from build123d import *

# Parameters (mm, degrees)
RESSALTO_EXTRUS_O1_DEPTH   = 285
CORTE_EXTRUS_O1_DEPTH      = 1
CORTE_EXTRUS_O1_DEPTH_BACK = 286


with BuildPart() as part:
    # Esboço1 → Ressalto-extrusão1 (new body)
    with BuildSketch(Plane.XY):
        Polygon((0.129363371, 0.000429576), (0.129363371, 50.000429576), (115.229363371, 50.000429576), (115.229363371, 0.000429576), (112.558897843, 0.0275034), (111.229363371, 41.700429576), (105.129363371, 41.700429576), (103.799966135, 0.000429576), (102.459761608, 0.000429576), (101.129363371, 41.700429576), (95.029363371, 41.700429576), (93.699966135, 0.000429576), (92.359761608, 0.000429576), (91.029363371, 41.700429576), (84.929363371, 41.700429576), (83.599966135, 0.000429576), (82.259761608, 0.000429576), (80.929363371, 41.700429576), (74.829363371, 41.700429576), (73.499966135, 0.000429576), (72.159761608, 0.000429576), (70.829363371, 41.700429576), (64.729363371, 41.700429576), (63.399966135, 0.000429576), (62.059761608, 0.000429576), (60.729363371, 41.700429576), (54.629363371, 41.700429576), (53.299966135, 0.000429576), (51.959761608, 0.000429576), (50.629363371, 41.700429576), (44.529363371, 41.700429576), (43.199966135, 0.000429576), (41.859761608, 0.000429576), (40.529363371, 41.700429576), (34.429363371, 41.700429576), (33.099966135, 0.000429576), (31.759761608, 0.000429576), (30.429363371, 41.700429576), (24.329363371, 41.700429576), (22.999966135, 0.000429576), (21.659761608, 0.000429576), (20.329363371, 41.700429576), (14.229363371, 41.700429576), (12.899966135, 0.000429576), (11.559761608, 0.000429576), (10.229363371, 41.700429576), (4.129363371, 41.700429576), (2.799966135, 0.000429576), align=None)
    extrude(amount=RESSALTO_EXTRUS_O1_DEPTH)

    # Esboço2 → Corte-extrusão1 (cut, two sides)
    with BuildSketch(Plane(origin=(0, 0, 0), x_dir=(-1, 0, 0), z_dir=(0, 0, -1))) as corte_extrus_o1_sk:
        Polygon((-104.72087071, 48.268772175), (-101.689781797, 46.518772175), (-102.689781797, 44.786721368), (-105.72087071, 46.536721368), (-108.513105078, 41.700429576), (-108.513105078, 0.000429576), (-115.229363371, 0.000429576), (-115.229363371, 50.000429576), (-103.74577832, 50.000429576), align=None)
        Polygon((-10.613175555, 48.268772175), (-8.881124748, 49.268772175), (-7.881124748, 47.536721368), (-9.613175555, 46.536721368), (-6.820941187, 41.700429576), (-6.820941187, 0), (0, 0), (-0.129363371, 50.000429576), (-11.612948422, 50.000429576), align=None)
    extrude(amount=CORTE_EXTRUS_O1_DEPTH, mode=Mode.SUBTRACT)
    extrude(corte_extrus_o1_sk.sketch, amount=-CORTE_EXTRUS_O1_DEPTH_BACK, mode=Mode.SUBTRACT)


solid = part.part
The listing builds one solid part. Answer for the finished solid, in the listing's coordinates (mm). Give positions to 0.01 mm unless a question says otherwise; leave off trailing zeros. Write each loop counter-clockwise with the first axis right and the second up, starting at its lowest first coordinate (ties: lowest second). Pieces come first, ordered by that corner, then holes.
1) Find the intervals of material crossed by L1, parallel to Y at x = 65, z = 233; L2, parallel to X at y = 42, z = 21, in increasing order.
2) Section B-B (x = 98) is taken. Write down the section's boundary in (y, z), and give its area (3 significant figures).
3) Given P1, Ø1.5, axis at x = 21, z = 68, coming from the -Y side; P2, Ø1.8, axis at x = 98.5, z = 204.5, coming from the -Y side; P3, Ø3, axis at y = 11.5, z = 144, coming from the +X side; P4, Ø8, axis at y = 31, z = 79, coming from the +X side, each flat-ended and moving along its own axis, determine where each tip first touches the part or whether it passes through.
4) Section A-A (y = 24) is taken. Count the separate pieces of the cut face and the enclosed holes in it, and give its area (3 significant figures).
5) For a pull along X with two mould halves and no side action, classify faces 1 (the face through (107.1, 44.15, 140.5)), 2 (the face through (58, 41.7, 141)) as pulls with the +X half, pulls with the -X half, needs draft (parallel to the pull), parting line crosses it, or undercut.
Response:
1. L1: y = 41.7 to 50
1. L2: x = 6.99 to 108.34
2. outline: (41.7, 0) - (50, 0) - (50, 285) - (41.7, 285) - close
2. area: 2,370 mm2
3. P1: stops at y = 0
3. P2: stops at y = 41.7
3. P3: stops at x = 104.21
3. P4: stops at x = 104.92
4. separate pieces: 10
4. enclosed holes: 0
4. area: 8,180 mm2
5. face 1: pulls with the +X half
5. face 2: undercut
